Input: part model. Units: mm. Frame: model coordinates. A direction names the side the tool comes from. Coordinates: 2 decimals unless noted, no trailing zeros. Write each loop counter-clockwise with the first axis right and the second up, starting at its lowest first coordinate (ties: lowest second). Pieces come first, ordered by that corner, then holes.
1) Section query B-B (y = 16.5). Output: boundary loops of the cut face in (x, z).
2) Section query D-D (z = 3.95). Output: boundary loops of the cut face in (x, y), then the cut area to 3 significant figures.
3) Set-up query: faces 1 (the flat face through (-5, 18, 0)), 2 (the flat face through (-20.75, 0, 4)), 3 (the flat face through (-21, -1.25, 3)). Return all of +Z, -Z, +X, -X, +Y, -Y with unobstructed straight access to the full face (end or side cutting, diameter ignored); none if empty.
4) Section query A-A (x = 0). Output: boundary loops of the cut face in (y, z).
5) Draft query along Y for faces 4 (the cylindrical face through (9.84, 15.43, 1.23)), 5 (the flat face through (-21, 1.25, 3)), 6 (the flat face through (-5, -18, 2.5)). Return one class per face: pulls with the +Y half, pulls with the -Y half, needs draft (parallel to the pull), parting line crosses it, or undercut.
6) Line query: L1, parallel to Y at x = 0, z = 1.7; L2, parallel to X at y = 7, z = 0.55 (3 decimals); L3, parallel to Y at x = -6.5, z = 0.4. Output: solid intervals per line, ascending.
7) Pin query (flat end, axial travel): pin 1 Ø0.8 at (x, z) = (-21, 2.5) entering from +Y; pin 2 Ø2 at (x, z) = (8, 3) entering from -Y; pin 3 Ø1.2 at (y, z) = (0.5, 4) entering from +X. Return the tip coordinate at first contact, or that it passes through.
8) Section query C-C (z = 1.2). Output: boundary loops of the cut face in (x, y).
from build123d import *

# Parameters (mm, degrees)
F0_R     = 20
F0_R_2   = 18.3
F1_DEPTH = 2.5
F3_DEPTH = 1.25


with BuildPart() as f1:
    # F0 (on Top) → F1 (new body)
    with BuildSketch(Plane.XY):
        Circle(F0_R)
        Circle(F0_R_2, mode=Mode.SUBTRACT)
    extrude(amount=F1_DEPTH)

    # F2 (on Front) → F3 (join, symmetric)
    with BuildSketch(Plane.XZ):
        Polygon((-20.75, 0), (-19.25, 0), (-19.25, 2.5), (-20.75, 2.5), (-20.75, 5), (-22.75, 5), (-22.75, 2), align=None)
    extrude(amount=F3_DEPTH, both=True)


solid = f1.part
Answer:
1. outline: (-11.3, 0) - (-7.91, 0) - (-7.91, 2.5) - (-11.3, 2.5) - close; (7.91, 0) - (11.3, 0) - (11.3, 2.5) - (7.91, 2.5) - close
2. outline: (-22.75, -1.25) - (-20.75, -1.25) - (-20.75, 1.25) - (-22.75, 1.25) - close
2. area: 5.00 mm2
3. face 1: -Z, +X, -X, +Y, -Y
3. face 2: +Z, +X, +Y, -Y
3. face 3: +Z, -Z, -X, -Y
4. outline: (-20, 0) - (-18.3, 0) - (-18.3, 2.5) - (-20, 2.5) - close; (18.3, 0) - (20, 0) - (20, 2.5) - (18.3, 2.5) - close
5. face 4: undercut
5. face 5: pulls with the +Y half
5. face 6: needs draft
6. L1: y = -20 to -18.3, 18.3 to 20
6. L2: x = -18.735 to -16.908, 16.908 to 18.735
6. L3: y = -18.91 to -17.11, 17.11 to 18.91
7. pin 1: stops at y = 1.25
7. pin 2: stops at y = -18.68
7. pin 3: stops at x = -20.75
8. outline: (-21.95, -1.25) - (-19.96, -1.25) arc R20 ccw (long way) to (-19.96, 1.25) - (-21.95, 1.25) - close; hole circle Ø36.6 at (0, 0)
